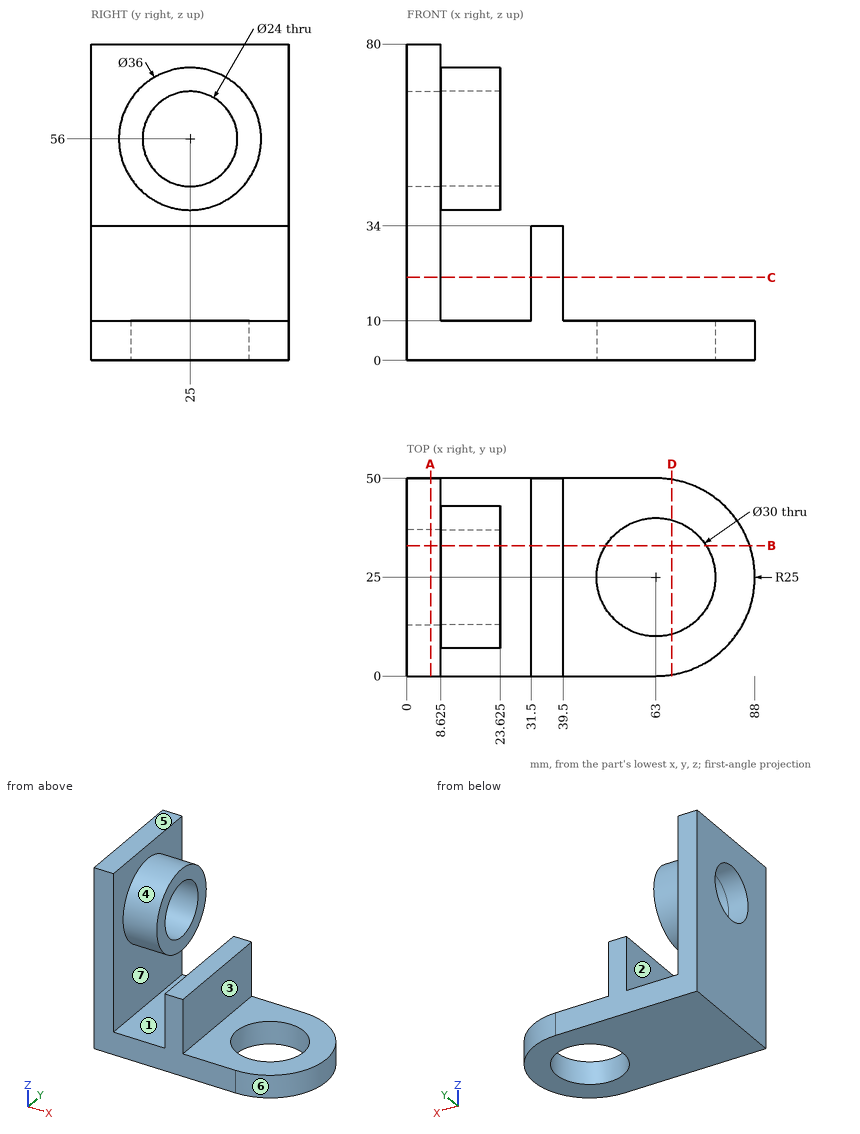
Design review of the part shown in the three views and the two pictorial views. Dimensions are in mm from the part's minimum x, y and z. A direction names the side the tool comes from. Round coordinates to 2 decimals unless told otherwise and drop trailing zeros. Write each loop counter-clockwise with the first axis right and the second up, starting at its lowest first coordinate (ties: lowest second). Pieces come first, ordered by that corner, then holes. Notation, with made-up numbers: (51, 40.25) -> (97, 40.25) arc R14 ccw to (97, 52.25) -> close; hole circle Ø2 at (10, -3.75). An arc over 180 degrees is marked (long way). Write item = value, one per line. Start each with the question number.
1) Take a section at B-B, the plane y = 33. State the section outline as (x, z) points (1 decimal).
2) Tool access review of the marked faces 1, 2 and 3: name each direction out of +Z, -Z, +X, -X, +Y, -Y from which nothing blocks a thin tool from reaching the whole face with its end or side.
3) Wall thickness on probe 1 along Z at (x, y) = (13, 25); probe 2 along X at (y, z) = (45, 17) (1 decimal); probe 3 along Z at (x, y) = (5, 25): over which ranges is each line inside the solid? List them lowest first. Write a range as from..to.
4) Clearance check with flat-ended pins moving along their axes: pin 1 (4 mm diameter, centred on x = 18, z = 39.5, fed in from +Y) (1 decimal); pin 2 (19 mm diameter, centred on y = 27.5, z = 24.5, fed in from +X); pin 3 (4 mm diameter, centred on x = 74.5, y = 10, fed in from +Z). State where each tip first meets the part, or that it passes through.
5) Mouldability with a two-part tool opening along Z and no side actions: class the marked faces 4, 5, 6 and 7 as +Z half, -Z half, draft (parallel to the pull), parting line (faces both ways), or undercut.
6) Take a section at D-D, the plane x = 67. State the section outline as (y, z) points, plus the area to 3 significant figures.
7) Take a section at A-A, the plane x = 6. State the section outline as (y, z) points, plus the area to 3 significant figures.
8) Take a section at C-C, the plane z = 21. State the section outline as (x, y) points (1 decimal).
Results list:
q1.outline = (0, 0) -> (50.3, 0) -> (50.3, 10) -> (39.5, 10) -> (39.5, 34) -> (31.5, 34) -> (31.5, 10) -> (8.6, 10) -> (8.6, 39.9) -> (23.6, 39.9) -> (23.6, 47.1) -> (0, 47.1) -> close; (0, 64.9) -> (23.6, 64.9) -> (23.6, 72.1) -> (8.6, 72.1) -> (8.6, 80) -> (0, 80) -> close; (75.7, 0) -> (86.7, 0) -> (86.7, 10) -> (75.7, 10) -> close
q2.face_1 = +Y, -Y
q2.face_2 = +Z, +Y, -Y
q2.face_3 = +Z, +X, +Y, -Y
q3.probe_1 = 0..10, 38..44, 68..74
q3.probe_2 = 0..8.6, 31.5..39.5
q3.probe_3 = 0..44, 68..80
q4.pin_1 = 35.7
q4.pin_2 = 39.5
q4.pin_3 = 10
q5.face_4 = undercut
q5.face_5 = +Z half
q5.face_6 = draft
q5.face_7 = undercut
q6.outline = (0.32, 0) -> (10.54, 0) -> (10.54, 10) -> (0.32, 10) -> close; (39.46, 0) -> (49.68, 0) -> (49.68, 10) -> (39.46, 10) -> close
q6.area = 204 mm²
q7.outline = (0, 0) -> (50, 0) -> (50, 80) -> (0, 80) -> close; hole circle Ø24 at (25, 56)
q7.area = 3,550 mm²
q8.outline = (0, 0) -> (8.6, 0) -> (8.6, 50) -> (0, 50) -> close; (31.5, 0) -> (39.5, 0) -> (39.5, 50) -> (31.5, 50) -> close
